Source: CAD feature listing. Evaluate the final solid. Frame: model axes, mm. Face numbers are marked on the shaded views. Give positions to 0.01 mm unless a question says otherwise; leave off trailing zeros. Loops run counter-clockwise (first coordinate to the right, second up) from the corner with the lowest first, then second, coordinate; pieces in that order, holes last. Notation, with made-up numbers: (-8.75, -3.75) - (44.25, -3.75) arc R21 ccw to (44.25, 0.25) - close; hole circle Ø11 at (-10, -38.5). An arc over 180 degrees is marked (long way). Write each question's results on one line, items separated by ' | '. Start each with the question number.
(1) Cut plane B-B on y = -515. Return the cut outline in (x, z), then the cut area to 3 significant figures.
(2) Pull-direction query (X, two-part tool) for the marked faces 1 and 2; classes: pulls with the +X half, pulls with the -X half, needs draft (parallel to the pull), parting line crosses it, or undercut.
(3) Material intervals for line 1 along Z through (x, y) = (-142.5, -1047); line 2 along Z through (x, y) = (-159, -1769); line 3 along Y through (x, z) = (50.5, -68.5), sorted ascending. Write a range as [from, to].
(4) Contact query for flat-ended pins moving along their axis: pin 1 (3.5 mm diameter, centred on x = -144, y = -745, fed in from +Z); pin 2 (8 mm diameter, centred on x = -190, z = 140, fed in from +Y); pin 3 (0.9 mm diameter, centred on x = -144, y = -667.5, fed in from -Z). Output: stop coordinate, or through.
(5) Cut plane A-A on y = -1610.5. Return the cut outline in (x, z).
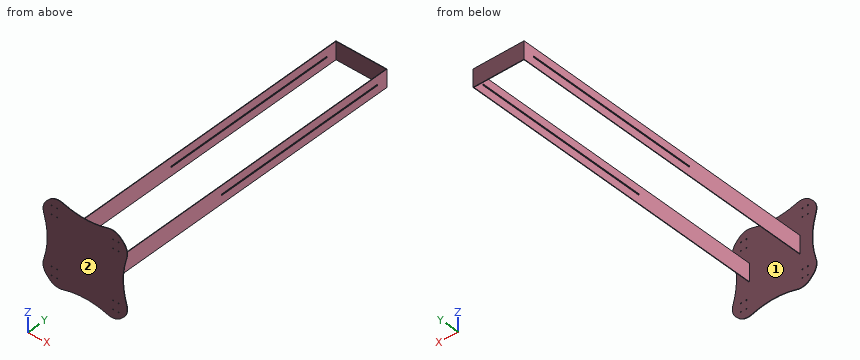
from build123d import *

# Parameters (mm, degrees)
SKETCH1_W           = 290
SKETCH1_H           = 3
BOSS_EXTRUDE1_DEPTH = 100
SKETCH2_W           = 3
SKETCH2_H           = 100
BOSS_EXTRUDE2_DEPTH = 1765.8
SKETCH5_W           = 8
SKETCH5_H           = 1000
CUT_EXTRUDE1_DEPTH  = 150
BOSS_EXTRUDE3_DEPTH = 3
FILLET1_R           = 75
SKETCH7_R           = 3
CUT_EXTRUDE2_DEPTH  = 10


with BuildPart() as part:
    # Sketch1 → Boss-Extrude1 (new body)
    with BuildSketch(Plane.XY):
        Rectangle(SKETCH1_W, SKETCH1_H)
    extrude(amount=-BOSS_EXTRUDE1_DEPTH)

    # Sketch2 → Boss-Extrude2 (add)
    with BuildSketch(Plane.XZ.offset(1.5)):
        with Locations((-143.5, -50)):
            Rectangle(SKETCH2_W, SKETCH2_H)
        with Locations((143.5, -50)):
            Rectangle(SKETCH2_W, SKETCH2_H)
    extrude(amount=BOSS_EXTRUDE2_DEPTH)

    # Sketch5 → Cut-Extrude1 (cut, symmetric)
    with BuildSketch(Plane(origin=(0, 0, 0), x_dir=(0, 0, -1), z_dir=(1, 0, 0))):
        with Locations((50, -558.5)):
            Rectangle(SKETCH5_W, SKETCH5_H)
    extrude(amount=CUT_EXTRUDE1_DEPTH, both=True, mode=Mode.SUBTRACT)

    # Sketch6 → Boss-Extrude3 (add)
    with BuildSketch(Plane.XZ.offset(1767.3)):
        with BuildLine():
            Line((-250, 120), (-170, 200))
            add(Edge.make_bspline(
                [(-170, 200), (0, 130), (170, 200)],
                knots=[0, 0, 0, 1, 1, 1], degree=2))
            Line((170, 200), (250, 120))
            add(Edge.make_bspline(
                [(250, 120), (180, -50), (250, -220)],
                knots=[0, 0, 0, 1, 1, 1], degree=2))
            Line((250, -220), (170, -300))
            add(Edge.make_bspline(
                [(-170, -300), (0, -230), (170, -300)],
                knots=[0, 0, 0, 1, 1, 1], degree=2))
            Line((-170, -300), (-250, -220))
            add(Edge.make_bspline(
                [(-250, 120), (-201.61826543, -7.179894106), (-205.048401237, -92.820105894), (-250, -220)],
                knots=[0, 0, 0, 0, 1, 1, 1, 1], degree=3))
        make_face()
    extrude(amount=BOSS_EXTRUDE3_DEPTH)

    # Fillet1
    fillet1_edges = [part.edges().sort_by_distance(p)[0] for p in [
        (250, -1768.8, 120),
        (-170, -1768.8, 200),
        (-250, -1768.8, 120),
        (-250, -1768.8, -220),
        (-170, -1768.8, -300),
        (170, -1768.8, -300),
        (250, -1768.8, -220),
        (170, -1768.8, 200),
    ]]
    fillet(fillet1_edges, radius=FILLET1_R)

    # Sketch7 → Cut-Extrude2 (cut)
    with BuildSketch(Plane.XZ.offset(1770.3)):
        with Locations(Location((-190, 140, 0), (0, 0, 270))):
            Circle(SKETCH7_R)
        with Locations(Location((-159, 140, 0), (0, 0, 270))):
            Circle(SKETCH7_R)
        with Locations(Location((-190, 92, 0), (0, 0, 270))):
            Circle(SKETCH7_R)
        with Locations(Location((-159, 92, 0), (0, 0, 270))):
            Circle(SKETCH7_R)
        with Locations(Location((190, 92, 0), (0, 0, 90))):
            Circle(SKETCH7_R)
        with Locations(Location((159, 92, 0), (0, 0, 90))):
            Circle(SKETCH7_R)
        with Locations(Location((159, 140, 0), (0, 0, 90))):
            Circle(SKETCH7_R)
        with Locations(Location((190, 140, 0), (0, 0, 90))):
            Circle(SKETCH7_R)
        with Locations(Location((159, -192, 0), (0, 0, 270))):
            Circle(SKETCH7_R)
        with Locations(Location((190, -192, 0), (0, 0, 270))):
            Circle(SKETCH7_R)
        with Locations(Location((190, -240, 0), (0, 0, 270))):
            Circle(SKETCH7_R)
        with Locations(Location((159, -240, 0), (0, 0, 270))):
            Circle(SKETCH7_R)
        with Locations(Location((-190, -192, 0), (0, 0, 90))):
            Circle(SKETCH7_R)
        with Locations(Location((-159, -192, 0), (0, 0, 90))):
            Circle(SKETCH7_R)
        with Locations(Location((-159, -240, 0), (0, 0, 90))):
            Circle(SKETCH7_R)
        with Locations(Location((-190, -240, 0), (0, 0, 90))):
            Circle(SKETCH7_R)
    extrude(amount=-CUT_EXTRUDE2_DEPTH, mode=Mode.SUBTRACT)


solid = part.part
Ans:
1) outline: (-145, -100) - (-142, -100) - (-142, -54) - (-145, -54) - close; (-145, -46) - (-142, -46) - (-142, 0) - (-145, 0) - close; (142, -100) - (145, -100) - (145, -54) - (142, -54) - close; (142, -46) - (145, -46) - (145, 0) - (142, 0) - close | area: 552 mm^2
2) face 1: undercut | face 2: needs draft
3) line 1: [-100, -54], [-46, 0] | line 2: [-287.86, -243], [-237, -195], [-189, 89], [95, 137], [143, 187.86] | line 3: [-1770.3, -1767.3], [-1.5, 1.5]
4) pin 1: z = 0 | pin 2: y = -1767.3 | pin 3: z = -100
5) outline: (-145, -100) - (-142, -100) - (-142, 0) - (-145, 0) - close; (142, -100) - (145, -100) - (145, 0) - (142, 0) - close
